Geometry check sheet. Reference: the model listing, model coordinates, mm. Face numbers are marked on the shaded views. Round coordinates to 2 decimals unless told otherwise and drop trailing zeros. One line per item, written item: value. Start each with the question number.
1. Scan lines: probe 1 along Y at (x, z) = (0, -2.9); probe 2 along Y at (x, z) = (-7, -2.75); probe 3 along X at (y, z) = (-6.5, -14). Record each from-to range of solid material in increasing order. Write a range as [from, to].
2. Release check for a two-part mould opening along X. For the marked faces 1, 2 and 3 record: pulls with the +X half, pulls with the -X half, needs draft (parallel to the pull), parting line crosses it, or undercut.
3. Depth check by flat-ended pin: P1, Ø4, axis at y = -12.5, z = -10.5, coming from the +X side; P2, Ø3, axis at x = -12.5, y = -7, coming from the -Z side; P3, Ø2, axis at x = 19.5, z = -7, coming from the -Y side; P4, Ø1.5, axis at x = -15.5, y = -5.5, coming from the +Z side. Enter the tip coordinate at first touch or a pass-through.
from build123d import *

# Parameters (mm, degrees)
SKETCH1_R        = 13.9175
BASENUT_DEPTH    = 28.6
ENDCHAMFER2_SIZE = 2.2825
LPATTERN10_COUNT = 9
LPATTERN10_PITCH = 2.739


with BuildPart() as part:
    # Sketch1 → BaseNut (new body)
    with BuildSketch(Plane.XY):
        Polygon((13.279056191, -23), (26.558112383, 0), (13.279056191, 23), (-13.279056191, 23), (-26.558112383, 0), (-13.279056191, -23), align=None)
        Circle(SKETCH1_R, mode=Mode.SUBTRACT)
    extrude(amount=-BASENUT_DEPTH)

    # Sketch2 → Chamfer1 (revolve, cut)
    with BuildSketch(Plane(origin=(15.04811501, 0, -16.706149795), x_dir=(0, 0, -1), z_dir=(0, 1, 0))):
        Polygon((9.839573063, 41.606227393), (11.893850205, 38.04811501), (11.893850205, 41.606227393), align=None)
    revolve(axis=Axis((0, 0, 7.016501752), (0, 0, -1)), mode=Mode.SUBTRACT)

    # Sketch6 → EndChamfer1 (revolve, cut)
    with BuildSketch(Plane(origin=(-9.197458863, 0, -10.252541137), x_dir=(0, 0, 1), z_dir=(0, 1, 0))):
        Polygon((-18.347458863, 23.114958863), (-18.347458863, 25.397458863), (-17.029656873, 23.114958863), align=None)
    revolve(axis=Axis((0, 0, 13.104863586), (0, 0, -1)), mode=Mode.SUBTRACT)

    # Sketch5 → Chamfer2 (revolve, cut)
    with BuildSketch(Plane(origin=(-14.793032735, 0, -16.96123207), x_dir=(0, 0, 1), z_dir=(0, 1, 0)), mode=Mode.PRIVATE) as chamfer2_sk:
        Polygon((16.96123207, 36.168032735), (16.96123207, 41.351145118), (13.968760741, 41.351145118), align=None)
    revolve(chamfer2_sk.sketch.rotate(Axis((0, 0, -39.536013381), (0, 0, 1)), 180), axis=Axis((0, 0, -39.536013381), (0, 0, 1)), mode=Mode.SUBTRACT)

    # EndChamfer2
    endchamfer2_edges = [part.edges().sort_by_distance(p)[0] for p in [
        (-13.9175, 0, 0),
    ]]
    chamfer(endchamfer2_edges, length=ENDCHAMFER2_SIZE)

    # Sketch7 → Cut-Revolve10 (revolve, cut)
    with BuildSketch(Plane(origin=(0, 0, 0), x_dir=(1, 0, 0), z_dir=(0, 1, 0))):
        Polygon((11.635, 28.423448011), (13.9175, 28.423448011), (15.894202984, 27.282198011), (13.9175, 26.140948011), (11.635, 26.140948011), align=None)
    cut_revolve10 = revolve(axis=Axis((0, 0, -48.618332322), (0, 0, 1)), mode=Mode.SUBTRACT)

    # LPattern10: Cut-Revolve10 ×9
    with Locations(*[(0, 0, i * LPATTERN10_PITCH) for i in range(1, LPATTERN10_COUNT)]):
        add(cut_revolve10, mode=Mode.SUBTRACT)


solid = part.part
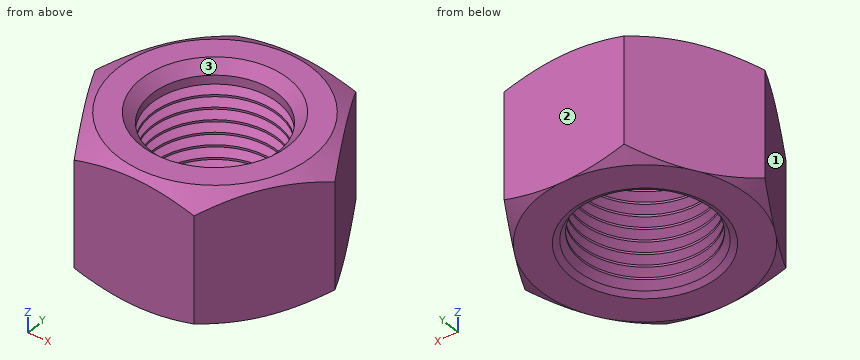
Result sheet:
1. probe 1: y = [-23, -13.92], [13.92, 23]
1. probe 2: y = [-23, -12.03], [12.03, 23]
1. probe 3: x = [-22.81, -13.72], [13.72, 22.81]
2. face 1: pulls with the -X half
2. face 2: needs draft
2. face 3: undercut
3. P1: stops at x = 20.5
3. P2: stops at z = -28.38
3. P3: stops at y = -13.96
3. P4: stops at z = 0
